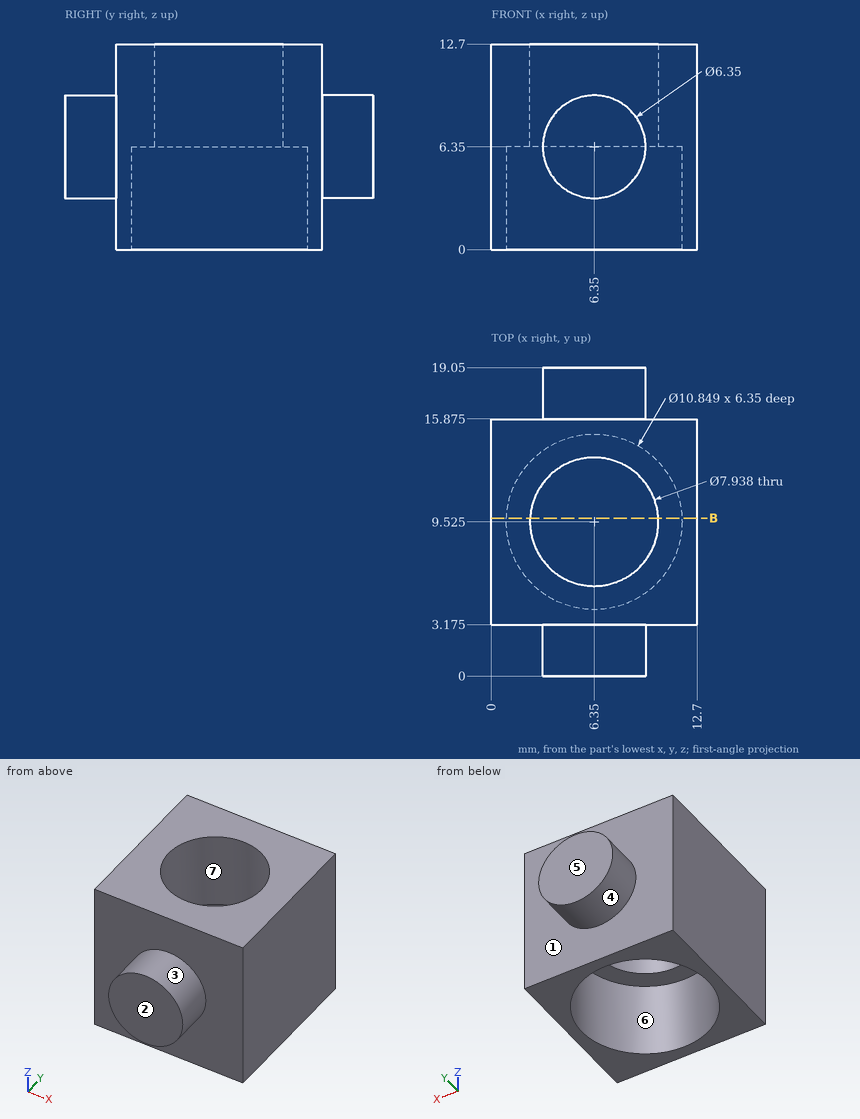
Check sheet for the drawn part. Datum: minimum x, y, z corner. Units: mm. A direction names the side the tool comes from. Round coordinates to 2 decimals unless told otherwise and drop trailing zeros. Loops run counter-clockwise (first coordinate to the right, second up) from the corner with the lowest first, then second, coordinate; pieces in that order, holes last. Notation, with made-up numbers: (74, -34.5) - (133, -34.5) arc R21 cw to (133, -3.5) - close; hole circle Ø5 at (-23.5, 82.25). An arc over 180 degrees is marked (long way). Answer as a JSON object with one key per item and string values. Group by question number.
Q1. Set-up check for the marked faces 1, 2 and 3: record each of +Z, -Z, +X, -X, +Y, -Y from which the full face is reachable in a straight line by a thin tool's end or side.
Q2. Sectioned sample at B-B, the plane y = 9.75. Enter the section's corners in (x, z).
Q3. Gauge pin test, flat ends, axial feed: P1, Ø5, axis at y = 13.5, z = 7, coming from the -X side; P2, Ø6.5, axis at x = 6.35, y = 9.525, coming from the +Z side; P3, Ø1.5, axis at x = 2, z = 7.5, coming from the +Y side (1 decimal). Record the tip position at first contact, or that the pin passes through.
Q4. Scan lines: line 1 along Y through (x, z) = (6.35, 4); line 2 along Y through (x, z) = (6.35, 11) (1 decimal); line 3 along Z through (x, y) = (6.5, 2). Record each from-to range of solid material in increasing order. Write a range as [from, to].
Q5. Mould release check, pull along Y, two halves, no side actions. Record for the marked faces 4, 5, 6 and 7: released by +Y, released by -Y, zero draft, split by the parting line, or undercut.
Solution:
{
 "1": {"face 1": "+Y", "face 2": "+Z, -Z, +X, -X, -Y", "face 3": "-Y"},
 "2": {"outline": "(0, 0) - (0.93, 0) - (0.93, 6.35) - (2.39, 6.35) - (2.39, 12.7) - (0, 12.7) - close; (10.31, 6.35) - (11.77, 6.35) - (11.77, 0) - (12.7, 0) - (12.7, 12.7) - (10.31, 12.7) - close"},
 "3": {"P1": "stops at x = 0", "P2": "passes through", "P3": "stops at y = 15.9"},
 "4": {"line 1": "y = [0, 4.1], [14.95, 19.05]", "line 2": "y = [3.2, 5.6], [13.5, 15.9]", "line 3": "z = [3.18, 9.52]"},
 "5": {"face 4": "zero draft", "face 5": "released by +Y", "face 6": "undercut", "face 7": "undercut"}
}
